Can you work these out from the drawing? Everything is in mm from the part's minimum corner. A direction names the side the tool comes from. Round coordinates to 2 decimals unless told otherwise and drop trailing zeros. Write each loop counter-clockwise with the first axis right and the second up, starting at its lowest first coordinate (ties: lowest second). Pieces come first, ordered by that corner, then holes. Notation, with made-up numbers: M 79,47 L 104,47 A19 cw 104,52 Z; hole C 81,5.25 d11. An arc over 180 degrees is marked long. Use a Markdown table: item, result. Add a question column.
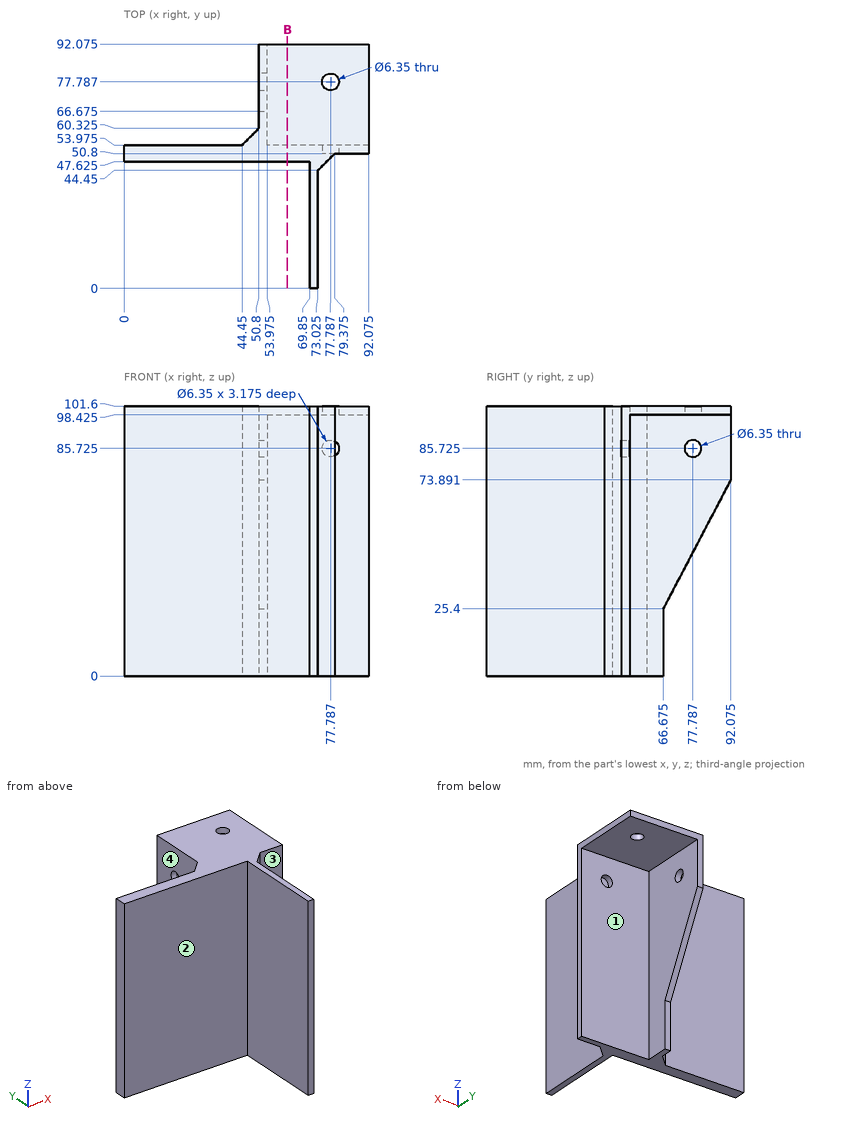
Item 1: On a 3-axis mill with a long thin cutter (end or side, diameter ignored), from which of +Z, -Z, +X, -X, +Y, -Y can I reach the whole of each face in a straight line? I mean the marked faces 1, 2, 3 and 4. Say none if no direction works.
Item 2: For pin 1 Ø4 at (x, z) = (89, 46) entering from -Y; pin 2 Ø22 at (x, z) = (28.5, 54.5) entering from +Y (1 decimal); pin 3 Ø6 at (x, z) = (35, 16) entering from -Y (1 decimal), each with a flat end and sliding along its axis, tell me the tip position at first contact or that it passes through.
Item 3: I need wall thicknesses on probe 1 along Y at (x, z) = (5.5, 4) (1 decimal); probe 2 along X at (y, z) = (62, 51.5) (1 decimal); probe 3 along Z at (x, y) = (62.5, 83) (1 decimal). Which ranges of each line are inside material? Lowest first, please. Write a range as from..to.
Item 4: Imagine slicing it at B-B on x = 61.5. List the corners of the cut face in (y, z) for me (1 decimal), plus the area to 3 significant figures.
The answers:
| question | item | result |
|---|---|---|
| 1 | face 1 | -Z, +X, +Y |
| 1 | face 2 | +Z, -Z, -X, -Y |
| 1 | face 3 | +Z, -Z, +X, -Y |
| 1 | face 4 | +Z, -Z, -X, +Y |
| 2 | pin 1 | y = 50.8 |
| 2 | pin 2 | y = 54 |
| 2 | pin 3 | y = 47.6 |
| 3 | probe 1 | 47.6..54 |
| 3 | probe 2 | 50.8..54 |
| 3 | probe 3 | 98.4..101.6 |
| 4 | outline | M 47.6,0 L 54,0 L 54,98.4 L 92.1,98.4 L 92.1,101.6 L 47.6,101.6 Z |
| 4 | area | 766 mm² |
